The listing builds one solid part. Answer for the finished solid, in the listing's coordinates (mm). Coordinates: 2 decimals unless noted, no trailing zeros. Order: outer loops, then holes, each group sorted by start corner. A loop starts at its lowest first (then second) coordinate and runs counter-clockwise, first axis right, second up. Notation, with made-up numbers: (56, -16) -> (74, -16) arc R30 ccw to (74, 13) -> close; hole circle Ø2 at (86, -20.5). An arc over 180 degrees is marked (long way). Put each result on its own line as item: value. Start each with the question number.
```python
from build123d import *

# Parameters (mm, degrees)
F1_DEPTH    = 5
F4_R        = 3
F5_DEPTH    = 5.001
F6_R        = 0.5
F7_T1_DEPTH = 5.5598599904
F9_R        = 4.8595532258
F9_R_2      = 3.1997304912
F10_DEPTH   = 0.5


# Not quite as in the source:
# - a fillet or chamfer that OpenCascade refuses, or shapes differently, is made with other operations: its cross-section is extruded or revolved along the edge and cut away or added


with BuildPart() as f1:
    # F0 (on Top) → F1 (new body)
    with BuildSketch(Plane.XY):
        Polygon((-2.8867513459, 5), (-5.7735026919, 0), (-2.8867513459, -5), (2.8867513459, -5), (5.7735026919, 0), (2.8867513459, 5), align=None)
    extrude(amount=F1_DEPTH)

    # F2 (on Front) → F3 (revolve, cut)
    with BuildSketch(Plane.XZ):
        Polygon((6, 1), (3.5, -0.285714148), (6, -0.285714148), align=None)
    revolve(axis=Axis((0, 0, 1.7616122495), (0, 0, 1)), mode=Mode.SUBTRACT)

    # F4 (on face) → F5 (cut, through all)
    with BuildSketch(Plane(origin=(0, 0, 0), x_dir=(1, 0, 0), z_dir=(0, 0, -1))):
        Circle(F4_R)
    extrude(amount=-F5_DEPTH, mode=Mode.SUBTRACT)

    # F6
    f6_edges = [f1.edges().sort_by_distance(p)[0] for p in [
        (-2.886751, 5, 2.941758),
    ]]
    fillet(f6_edges, radius=F6_R)

    # F7: fillet of radius 0.5 on 5 edges, made by hand

    # F7_s2 → F7_t1 (cut)
    with BuildSketch(Plane.XY.offset(0.1618278461)):
        with BuildLine():
            ThreePointArc((-5.6291651246, 0.25), (-5.6961524227, 0), (-5.6291651246, -0.25))
            Line((-5.6291651246, -0.25), (-5.7735026919, 0))
            Line((-5.7735026919, 0), (-5.6291651246, 0.25))
        make_face()
        with BuildLine():
            ThreePointArc((-3.0310889132, -4.75), (-2.8480762114, -4.9330127019), (-2.5980762114, -5))
            Line((-2.5980762114, -5), (-2.8867513459, -5))
            Line((-2.8867513459, -5), (-3.0310889132, -4.75))
        make_face()
        with BuildLine():
            ThreePointArc((2.5980762114, -5), (2.8480762114, -4.9330127019), (3.0310889132, -4.75))
            Line((3.0310889132, -4.75), (2.8867513459, -5))
            Line((2.8867513459, -5), (2.5980762114, -5))
        make_face()
        with BuildLine():
            ThreePointArc((5.6291651246, 0.25), (5.6961524227, 0), (5.6291651246, -0.25))
            Line((5.6291651246, -0.25), (5.7735026919, 0))
            Line((5.7735026919, 0), (5.6291651246, 0.25))
        make_face()
        with BuildLine():
            ThreePointArc((2.5980762114, 5), (2.8480762114, 4.9330127019), (3.0310889132, 4.75))
            Line((3.0310889132, 4.75), (2.8867513459, 5))
            Line((2.8867513459, 5), (2.5980762114, 5))
        make_face()
    extrude(amount=F7_T1_DEPTH, mode=Mode.SUBTRACT)

    # F9 (on face) → F10 (join)
    with BuildSketch(Plane.XY.offset(5)):
        Circle(F9_R)
        Circle(F9_R_2, mode=Mode.SUBTRACT)
    extrude(amount=F10_DEPTH)


solid = f1.part
```
(1) The part is cut by section A-A on x = 0. Determine the outline of the cut face in (y, z), plus the area to 3 significant figures.
(2) For a pull along X with two mould halves and no side action, classify faces 1 (the flat face through (-5, -1, 5)), 2 (the cylindrical face through (2.61, 4.1, 5.25)), 3 (the cylindrical face through (2.956, -1.226, 5.246)) as released by +X, released by -X, zero draft, split by the parting line, or undercut.
(3) The part is cut by section C-C on z = 4.6. Determine the outline of the cut face in (x, y).
(4) Each of these flat-tipped pins is pushed along its axis until it touches: P1, Ø5, axis at x = -1, y = 1.5, coming from the +Z side; P2, Ø1, axis at y = -3.5, z = 2.5, coming from the -X side; P3, Ø1.9, axis at x = -1.5, y = -1.5, coming from the +Z side. Where does it stop, or does it pass through?
(5) Find the intervals of material crossed by L1, parallel to Y at x = 0, z = 1.8; L2, parallel to Y at x = 0, z = 5.2; L3, parallel to X at y = 0, z = 1.1, in increasing order.
(6) The part is cut by section B-B on y = 0. Determine the outline of the cut face in (x, z).
Worked out:
1. outline: (-5, 0.49) -> (-4.06, 0) -> (-3, 0) -> (-3, 5) -> (-3.2, 5) -> (-3.2, 5.5) -> (-4.86, 5.5) -> (-4.86, 5) -> (-5, 5) -> close; (3, 0) -> (4.06, 0) -> (5, 0.49) -> (5, 5) -> (4.86, 5) -> (4.86, 5.5) -> (3.2, 5.5) -> (3.2, 5) -> (3, 5) -> close
1. area: 21.2 mm2
2. face 1: zero draft
2. face 2: split by the parting line
2. face 3: undercut
3. outline: (-5.63, -0.25) -> (-3.03, -4.75) arc R0.5 ccw to (-2.6, -5) -> (2.6, -5) arc R0.5 ccw to (3.03, -4.75) -> (5.63, -0.25) arc R0.5 ccw to (5.63, 0.25) -> (3.03, 4.75) arc R0.5 ccw to (2.6, 5) -> (-2.6, 5) arc R0.5 ccw to (-3.03, 4.75) -> (-5.63, 0.25) arc R0.5 ccw to start; hole circle Ø6 at (0, 0)
4. P1: z = 5.5
4. P2: x = -4.04
4. P3: z = 5
5. L1: -5 to -3, 3 to 5
5. L2: -4.86 to -3.2, 3.2 to 4.86
5. L3: -5.7 to -3, 3 to 5.7
6. outline: (-5.7, 0.84) -> (-4.06, 0) -> (-3, 0) -> (-3, 5) -> (-3.2, 5) -> (-3.2, 5.5) -> (-4.86, 5.5) -> (-4.86, 5) -> (-5.7, 5) -> close; (3, 0) -> (4.06, 0) -> (5.7, 0.84) -> (5.7, 5) -> (4.86, 5) -> (4.86, 5.5) -> (3.2, 5.5) -> (3.2, 5) -> (3, 5) -> close
